Design review of the part built by this model. Coordinates are the model's own, in mm. Give positions to 0.01 mm unless a question says otherwise; leave off trailing zeros. Order: outer loops, then holes, each group sorted by start corner. A loop starts at its lowest first (then second) coordinate and runs counter-clockwise, first axis right, second up. Notation, with made-up numbers: M -31,-8 L 26,-8 A15 cw 26,3 Z; hole C -18,-34 d9. An arc over 180 degrees is marked long. Put each result on its own line as item: value. Start each with the question number.
from build123d import *

# Parameters (mm, degrees)
F1_DEPTH = 3
F2_R     = 3
F3_R     = 1.5
F4_DEPTH = 3


with BuildPart() as f1:
    # F0 (on Top) → F1 (new body)
    with BuildSketch(Plane.XY):
        Polygon((0, 75.055535), (-65, -37.527767), (65, -37.527767), align=None)
    extrude(amount=F1_DEPTH)

    # F2
    f2_edges = [f1.edges().sort_by_distance(p)[0] for p in [
        (-65, -37.527767, 1.5),
        (65, -37.527767, 1.5),
        (0, 75.055535, 1.5),
    ]]
    fillet(f2_edges, radius=F2_R)

    # F3 (on face) → F4 (cut, through all)
    with BuildSketch(Plane.XY.offset(3)):
        Circle(F3_R)
    extrude(amount=-F4_DEPTH, mode=Mode.SUBTRACT)


solid = f1.part
1. Consider section C-C on z = 2.05. Give the boundary of the cut face in (x, y), then the cut area to 3 significant figures.
2. Insertion check: pin 1 (2.5 mm diameter, centred on x = 0, y = 0, fed in from +Z); pin 2 (1.5 mm diameter, centred on y = 0.5, z = 1.5, fed in from +X); pin 3 (1.5 mm diameter, centred on y = -10, z = 2.5, fed in from +X); pin 4 (1.5 mm diameter, centred on x = -15.5, z = 2.5, fed in from +Y). Each pin has a flat end and moves straight along its axis. Give the tip position at first contact, or say it passes through.
3. Consider section A-A on x = 0. Give the boundary of the cut face in (y, z), then the cut area to 3 significant figures.
4. Consider section B-B on y = 0. Give the boundary of the cut face in (x, z).
5. Consider section D-D on x = 50.5. Give the boundary of the cut face in (y, z).
6. To check wall thickness, follow probe 1 along Y at (x, z) = (0, 1.65); probe 2 along X at (y, z) = (15, 2.35); probe 3 along Y at (x, z) = (-48.5, 0.55). State the ranges of each line that lie inside material, in increasing order.
7. The part is to be moulded in two halves that separate along X. For faces 1 (the flat face through (-1, 6, 0)), 2 (the cylindrical face through (-1.5, 0.07, 1.52)), 3 (the flat face through (-32.08, 19.49, 1.48)), say which applies: +X half, -X half, draft (parallel to the pull), parting line (faces both ways), or undercut.
Returned:
1. outline: M -62.4,-33.03 A3 ccw -59.8,-37.53 L 59.8,-37.53 A3 ccw 62.4,-33.03 L 2.6,70.56 A3 ccw -2.6,70.56 Z; hole C 0,0 d3
1. area: 7,290 mm2
2. pin 1: passes through
2. pin 2: stops at x = 43.48
2. pin 3: stops at x = 49.54
2. pin 4: stops at y = 49.51
3. outline: M -37.53,0 L -1.5,0 L -1.5,3 L -37.53,3 Z; M 1.5,0 L 72.06,0 L 72.06,3 L 1.5,3 Z
3. area: 320 mm2
4. outline: M -43.33,0 L -1.5,0 L -1.5,3 L -43.33,3 Z; M 1.5,0 L 43.33,0 L 43.33,3 L 1.5,3 Z
5. outline: M -37.53,0 L -12.41,0 L -12.41,3 L -37.53,3 Z
6. probe 1: y = -37.53 to -1.5, 1.5 to 72.06
6. probe 2: x = -34.67 to 34.67
6. probe 3: y = -37.53 to -8.95
7. face 1: draft
7. face 2: undercut
7. face 3: -X half
